```python
from build123d import *

# Parameters (mm, degrees)
SKETCH_1_R      = 1.5
SKETCH_1_R_2    = 11
EXTRUDE_1_DEPTH = 3
EXTRUDE_2_DEPTH = 3
RIB_2_REACH     = 81.244
SKETCH_4_WALL_W = 177.006790998
SKETCH_4_WALL_H = 3


with BuildPart() as part:
    # 草图1 → 凸台-拉伸1 (new body)
    with BuildSketch(Plane(origin=(0, 0, 0), x_dir=(1, 0, 0), z_dir=(0, 1, 0))):
        Polygon((-25, -23.05), (25, -23.05), (25, 23.05), (19.6, 28.45), (-19.6, 28.45), (-25, 23.05), align=None)
        with Locations(Location((-15.5, 22.95, 0), (0, 0, 270))):
            Circle(SKETCH_1_R, mode=Mode.SUBTRACT)
        with Locations(Location((15.5, 22.95, 0), (0, 0, 90))):
            Circle(SKETCH_1_R, mode=Mode.SUBTRACT)
        with Locations(Location((-15.5, -8.05, 0), (0, 0, 270))):
            Circle(SKETCH_1_R, mode=Mode.SUBTRACT)
        with Locations(Location((15.5, -8.05, 0), (0, 0, 90))):
            Circle(SKETCH_1_R, mode=Mode.SUBTRACT)
        with Locations(Location((0, 7.45, 0), (0, 0, 270))):
            Circle(SKETCH_1_R_2, mode=Mode.SUBTRACT)
    extrude(amount=EXTRUDE_1_DEPTH)

    # 草图3 → 凸台-拉伸2 (add)
    with BuildSketch(Plane.XY.offset(23.05)):
        Polygon((25, 0), (-25, 0), (-25, 48.1), (-19.6, 54.5), (19.6, 54.5), (25, 48.1), align=None)
        with BuildLine():
            Line((-11.85, 42.35), (-11.85, 15.15))
            ThreePointArc((-11.85, 15.15), (-15, 12), (-18.15, 15.15))
            Line((-18.15, 15.15), (-18.15, 42.35))
            ThreePointArc((-18.15, 42.35), (-15, 45.5), (-11.85, 42.35))
        make_face(mode=Mode.SUBTRACT)
        with BuildLine():
            Line((11.85, 42.35), (11.85, 15.15))
            ThreePointArc((11.85, 15.15), (15, 12), (18.15, 15.15))
            Line((18.15, 15.15), (18.15, 42.35))
            ThreePointArc((18.15, 42.35), (15, 45.5), (11.85, 42.35))
        make_face(mode=Mode.SUBTRACT)
    extrude(amount=-EXTRUDE_2_DEPTH)

    # 草图4 wall → 筋2 (add, up to next)
    with BuildSketch(Plane(origin=(-25, 8.840091802, 14.209908198), x_dir=(0, -0.707106781187, -0.707106781187), z_dir=(0, -0.707106781187, 0.707106781187)), mode=Mode.PRIVATE) as rib_2_sk1:
        with Locations((0, 1.5)):
            Rectangle(SKETCH_4_WALL_W, SKETCH_4_WALL_H)
    rib_2_tool1 = extrude(rib_2_sk1.sketch, amount=RIB_2_REACH, mode=Mode.PRIVATE) - part.part
    rib_2 = rib_2_tool1.solids().sort_by_distance((-25, 8.840091802, 14.209908198))[0]
    add(rib_2)

    # 镜向1: 筋2 across plane
    add(rib_2.mirror(Plane(origin=(0, 0, 0), x_dir=(0, 0, 1), z_dir=(1, 0, 0))))


solid = part.part
```
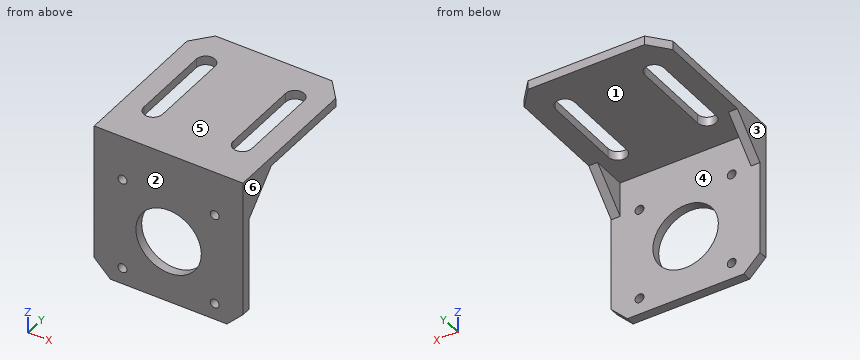
CAD build for the part. Positions are in the model's coordinates, mm. Face numbers are marked on the shaded views. A direction names the side the tool comes from. Round coordinates to 2 decimals unless told otherwise and drop trailing zeros. Loops run counter-clockwise (first coordinate to the right, second up) from the corner with the lowest first, then second, coordinate; pieces in that order, holes last. Notation, with made-up numbers: M 2,70.5 L 8,70.5 A32 ccw 8,106.5 Z; hole C 34.5,-33 d9. An arc over 180 degrees is marked long. Return JSON: item names as keys, results as strings. Group by question number.
(1) Saw through at C-C, the plane x = 0. List the corners of the cut face in (y, z), and give its area (3 significant figures).
(2) Mould opens along X. For the marked faces 3, 4, 5 and 6 say: +X half, -X half, draft (parallel to the pull), parting line (faces both ways), or undercut.
(3) Tool access for the marked faces 1 and 2: list every direction of +Z, -Z, +X, -X, +Y, -Y with a clear straight run to the whole face (end or side of a thin tool).
(4) Saw through at B-B, the plane z = -7.45. List the corners of the cut face in (x, y), and give its area (3 significant figures).
(5) Saw through at D-D, the plane x = 15.5. List the corners of the cut face in (y, z).
(6) Saw through at A-A, the plane y = 24.5. List the corners of the cut face in (x, z).
(7) Wall check: probe 1 along Z at (x, y) = (15.5, 0.75); probe 2 along X at (y, z) = (1.55, 8.05); probe 3 along Y at (x, z) = (-22, -7). Give the ranges that are in metal, low to high. Write a range as [from, to].
(8) Drop flat-ended pins along their axis: P1, Ø4, axis at x = -15.5, z = 8.05, coming from the +Y side; P2, Ø12, axis at x = 12.5, y = 29.5, coming from the -Z side. Give the stop position or say it passes through.
Answer list:
{
 "1": {"outline": "M 0,-28.45 L 3,-28.45 L 3,-18.45 L 0,-18.45 Z; M 0,3.55 L 3,3.55 L 3,20.05 L 54.5,20.05 L 54.5,23.05 L 0,23.05 Z", "area": "243 mm2"},
 "2": {"face 3": "-X half", "face 4": "undercut", "face 5": "draft", "face 6": "+X half"},
 "3": {"face 1": "-Z, +Y", "face 2": "+Z, -Z, +X, -X, -Y"},
 "4": {"outline": "M -25,0 L -11,0 L -11,3 L -25,3 Z; M 11,0 L 25,0 L 25,3 L 11,3 Z", "area": "84.0 mm2"},
 "5": {"outline": "M 0,-28.45 L 3,-28.45 L 3,-24.45 L 0,-24.45 Z; M 0,-21.45 L 3,-21.45 L 3,6.55 L 0,6.55 Z; M 0,9.55 L 3,9.55 L 3,20.05 L 12.04,20.05 L 12.04,23.05 L 0,23.05 Z; M 45.46,20.05 L 54.5,20.05 L 54.5,23.05 L 45.46,23.05 Z"},
 "6": {"outline": "M -25,20.05 L -18.15,20.05 L -18.15,23.05 L -25,23.05 Z; M -11.85,20.05 L 11.85,20.05 L 11.85,23.05 L -11.85,23.05 Z; M 18.15,20.05 L 25,20.05 L 25,23.05 L 18.15,23.05 Z"},
 "7": {"probe 1": "[-28.45, -24.45], [-21.45, 6.55], [9.55, 23.05]", "probe 2": "[-25, -17], [-14, 14], [17, 25]", "probe 3": "[0, 3]"},
 "8": {"P1": "y = 3", "P2": "z = 20.05"}
}
